Could you check a few things on this model? Use its own coordinates, in mm. A direction names the side the tool comes from. Coordinates: 2 decimals unless noted, no trailing zeros. Loops run counter-clockwise (first coordinate to the right, second up) from the corner with the lowest first, then second, coordinate; pieces in that order, holes last. Notation, with made-up numbers: M 87.25,57 L 102.25,57 A19 cw 102.25,65 Z; hole C 77.25,-36 d3. An arc over 180 degrees is marked long. Return JSON: item names as keys, results as strings. Group by question number.
from build123d import *

# Parameters (mm, degrees)
SKETCH_1_W           = 180
SKETCH_1_H           = 60
SKETCH_1_R           = 11
SKETCH_1_R_2         = 1.5
EXTRUDE_3_DEPTH      = 5
SKETCH_2_W           = 10
SKETCH_2_H           = 20
EXTRUDE_4_DEPTH      = 20
SKETCH_4_R           = 4
CUT_EXTRUDE_1_DEPTH  = 20
SKETCH_8_W           = 3
SKETCH_8_H           = 20
CUT_EXTRUDE_4_DEPTH  = 10
SKETCH_10_W          = 14
SKETCH_10_H          = 20
EXTRUDE_5_DEPTH      = 10
SKETCH_9_R           = 4
CUT_EXTRUDE_5_DEPTH  = 10
SKETCH_12_W          = 13.5
SKETCH_12_H          = 20
CUT_EXTRUDE_6_DEPTH  = 10
SKETCH_15_W          = 1
SKETCH_15_H          = 20
CUT_EXTRUDE_7_DEPTH  = 10
FILLET_5_R           = 5
SKETCH_21_W          = 10
SKETCH_21_H          = 18
EXTRUDE_6_DEPTH      = 20
SKETCH_25_W          = 11.311173877
SKETCH_25_H          = 1.5
CUT_EXTRUDE_10_DEPTH = 20
SKETCH_37_W          = 10
SKETCH_37_H          = 20
EXTRUDE_9_DEPTH      = 6
SKETCH_38_W          = 10
SKETCH_38_H          = 20
CUT_EXTRUDE_12_DEPTH = 6
SKETCH_39_R          = 4
CUT_EXTRUDE_13_DEPTH = 144.937604561
FILLET_10_R          = 8
SKETCH_41_R          = 1.5
CUT_EXTRUDE_14_DEPTH = 10
SKETCH_42_R          = 11.5
CUT_EXTRUDE_15_DEPTH = 10
SKETCH_43_R          = 1.691985253
CUT_EXTRUDE_16_DEPTH = 10
SKETCH_44_R          = 4.5
CUT_EXTRUDE_17_DEPTH = 10
CUT_EXTRUDE_18_DEPTH = 10


with BuildPart() as part:
    # 스케치1 → 보스-돌출3 (new body)
    with BuildSketch(Plane(origin=(0, 0, 0), x_dir=(1, 0, 0), z_dir=(0, 1, 0))):
        with Locations((36.632340007, -1.742375967)):
            Rectangle(SKETCH_1_W, SKETCH_1_H)
        with Locations(Location((105.632340007, 7.257624033, 0), (0, 0, 270))):
            Circle(SKETCH_1_R, mode=Mode.SUBTRACT)
        with Locations(Location((90.132340007, 22.757624033, 0), (0, 0, 270))):
            Circle(SKETCH_1_R_2, mode=Mode.SUBTRACT)
        with Locations(Location((121.132340007, 22.757624033, 0), (0, 0, 270))):
            Circle(SKETCH_1_R_2, mode=Mode.SUBTRACT)
        with Locations(Location((90.132340007, -8.242375967, 0), (0, 0, 270))):
            Circle(SKETCH_1_R_2, mode=Mode.SUBTRACT)
        with Locations(Location((121.132340007, -8.242375967, 0), (0, 0, 270))):
            Circle(SKETCH_1_R_2, mode=Mode.SUBTRACT)
        with Locations(Location((-32.617755763, 4.712595626, 0), (0, 0, 270))):
            Circle(SKETCH_1_R_2, mode=Mode.SUBTRACT)
        with Locations(Location((-45.654401225, 19.548720133, 0), (0, 0, 270))):
            Circle(SKETCH_1_R_2, mode=Mode.SUBTRACT)
        with Locations(Location((-45.654401225, -10.123528882, 0), (0, 0, 270))):
            Circle(SKETCH_1_R_2, mode=Mode.SUBTRACT)
    extrude(amount=EXTRUDE_3_DEPTH)

    # 스케치2 → 보스-돌출4 (add)
    with BuildSketch(Plane(origin=(0, 5, 0), x_dir=(1, 0, 0), z_dir=(0, 1, 0))):
        with Locations((79.782459712, 8.257624033)):
            Rectangle(SKETCH_2_W, SKETCH_2_H)
    extrude(amount=EXTRUDE_4_DEPTH)

    # 스케치4 → 컷-돌출1 (cut)
    with BuildSketch(Plane.ZY.offset(-74.782459712)):
        with Locations((-8.257624033, 15)):
            Circle(SKETCH_4_R)
    extrude(amount=-CUT_EXTRUDE_1_DEPTH, mode=Mode.SUBTRACT)

    # 스케치8 → 컷-돌출4 (cut)
    with BuildSketch(Plane(origin=(84.782459712, 0, 0), x_dir=(0, 0, -1), z_dir=(1, 0, 0))):
        with Locations((16.757624033, 15)):
            Rectangle(SKETCH_8_W, SKETCH_8_H)
        with Locations((-0.242375967, 15)):
            Rectangle(SKETCH_8_W, SKETCH_8_H)
    extrude(amount=-CUT_EXTRUDE_4_DEPTH, mode=Mode.SUBTRACT)

    # 스케치10 → 보스-돌출5 (add)
    with BuildSketch(Plane(origin=(84.782459712, 0, 0), x_dir=(0, 0, -1), z_dir=(1, 0, 0))):
        with Locations((-5.242375967, 15)):
            Rectangle(SKETCH_10_W, SKETCH_10_H)
    extrude(amount=-EXTRUDE_5_DEPTH)

    # 스케치9 → 컷-돌출5 (cut)
    with BuildSketch(Plane(origin=(84.782459712, 0, 0), x_dir=(0, 0, -1), z_dir=(1, 0, 0))):
        with Locations((-5.242375967, 15)):
            Circle(SKETCH_9_R)
    extrude(amount=-CUT_EXTRUDE_5_DEPTH, mode=Mode.SUBTRACT)

    # 스케치12 → 컷-돌출6 (cut)
    with BuildSketch(Plane(origin=(84.782459712, 0, 0), x_dir=(0, 0, -1), z_dir=(1, 0, 0))):
        with Locations((8.507624033, 15)):
            Rectangle(SKETCH_12_W, SKETCH_12_H)
    extrude(amount=-CUT_EXTRUDE_6_DEPTH, mode=Mode.SUBTRACT)

    # 스케치15 → 컷-돌출7 (cut)
    with BuildSketch(Plane(origin=(84.782459712, 0, 0), x_dir=(0, 0, -1), z_dir=(1, 0, 0))):
        with Locations((1.257624033, 15)):
            Rectangle(SKETCH_15_W, SKETCH_15_H)
    extrude(amount=-CUT_EXTRUDE_7_DEPTH, mode=Mode.SUBTRACT)

    # 필렛5
    fillet_5_edges = [part.edges().sort_by_distance(p)[0] for p in [
        (79.782459712, 25, -0.757624033),
        (79.782459712, 25, 12.242375967),
    ]]
    fillet(fillet_5_edges, radius=FILLET_5_R)

    # 스케치21 → 보스-돌출6 (add)
    with BuildSketch(Plane(origin=(0, 5, 0), x_dir=(1, 0, 0), z_dir=(0, 1, 0))):
        with Locations((79.782459712, -5.742375967)):
            Rectangle(SKETCH_21_W, SKETCH_21_H)
    extrude(amount=EXTRUDE_6_DEPTH)

    # 스케치25 → 컷-돌출10 (cut)
    with BuildSketch(Plane(origin=(0, 5, 0), x_dir=(1, 0, 0), z_dir=(0, 1, 0))):
        with Locations((79.126872773, 2.507624033)):
            Rectangle(SKETCH_25_W, SKETCH_25_H)
    extrude(amount=CUT_EXTRUDE_10_DEPTH, mode=Mode.SUBTRACT)

    # 스케치37 → 보스-돌출9 (add)
    with BuildSketch(Plane.XY.offset(14.742375967)):
        with Locations((79.782459712, 15)):
            Rectangle(SKETCH_37_W, SKETCH_37_H)
    extrude(amount=EXTRUDE_9_DEPTH)

    # 스케치38 → 컷-돌출12 (cut)
    with BuildSketch(Plane(origin=(0, 0, -1.757624033), x_dir=(-1, 0, 0), z_dir=(0, 0, -1))):
        with Locations((-79.782459712, 15)):
            Rectangle(SKETCH_38_W, SKETCH_38_H)
    extrude(amount=-CUT_EXTRUDE_12_DEPTH, mode=Mode.SUBTRACT)

    # 스케치39 → 컷-돌출13 (cut, through all)
    with BuildSketch(Plane(origin=(84.782459712, 0, 0), x_dir=(0, 0, -1), z_dir=(1, 0, 0))):
        with Locations((-11.742375967, 15)):
            Circle(SKETCH_39_R)
    extrude(amount=-CUT_EXTRUDE_13_DEPTH, mode=Mode.SUBTRACT)

    # 필렛10
    fillet_10_edges = [part.edges().sort_by_distance(p)[0] for p in [
        (79.782459712, 25, 20.742375967),
        (79.782459712, 5, 20.742375967),
        (79.782459712, 25, 4.242375967),
    ]]
    fillet(fillet_10_edges, radius=FILLET_10_R)

    # 스케치41 → 컷-돌출14 (cut)
    with BuildSketch(Plane(origin=(0, 5, 0), x_dir=(1, 0, 0), z_dir=(0, 1, 0))):
        with Locations(Location((-16.145477704, -6.751246634, 0), (0, 0, 270))):
            Circle(SKETCH_41_R)
        with Locations(Location((-16.145477704, 11.864366715, 0), (0, 0, 270))):
            Circle(SKETCH_41_R)
        with Locations(Location((0.854522296, 11.864366715, 0), (0, 0, 270))):
            Circle(SKETCH_41_R)
        with Locations(Location((0.854522296, -6.751246634, 0), (0, 0, 270))):
            Circle(SKETCH_41_R)
        with Locations(Location((17.854522296, 11.864366715, 0), (0, 0, 270))):
            Circle(SKETCH_41_R)
        with Locations(Location((17.854522296, -6.751246634, 0), (0, 0, 270))):
            Circle(SKETCH_41_R)
        with Locations(Location((34.854522296, 11.864366715, 0), (0, 0, 270))):
            Circle(SKETCH_41_R)
        with Locations(Location((34.854522296, -6.751246634, 0), (0, 0, 270))):
            Circle(SKETCH_41_R)
        with Locations(Location((51.854522296, 11.864366715, 0), (0, 0, 270))):
            Circle(SKETCH_41_R)
        with Locations(Location((51.854522296, -6.751246634, 0), (0, 0, 270))):
            Circle(SKETCH_41_R)
        with Locations(Location((68.854522296, 11.864366715, 0), (0, 0, 270))):
            Circle(SKETCH_41_R)
        with Locations(Location((68.854522296, -6.751246634, 0), (0, 0, 270))):
            Circle(SKETCH_41_R)
    extrude(amount=-CUT_EXTRUDE_14_DEPTH, mode=Mode.SUBTRACT)

    # 스케치42 → 컷-돌출15 (cut)
    with BuildSketch(Plane(origin=(0, 5, 0), x_dir=(1, 0, 0), z_dir=(0, 1, 0))):
        with Locations(Location((105.632340007, 7.257624033, 0), (0, 0, 270))):
            Circle(SKETCH_42_R)
    extrude(amount=-CUT_EXTRUDE_15_DEPTH, mode=Mode.SUBTRACT)

    # 스케치43 → 컷-돌출16 (cut)
    with BuildSketch(Plane(origin=(0, 0, 4.242375967), x_dir=(-1, 0, 0), z_dir=(0, 0, -1))):
        with Locations((-79.782459712, 14.121740896)):
            Circle(SKETCH_43_R)
    extrude(amount=-CUT_EXTRUDE_16_DEPTH, mode=Mode.SUBTRACT)

    # 스케치44 → 컷-돌출17 (cut)
    with BuildSketch(Plane.ZY.offset(-74.782459712)):
        with Locations((11.742375967, 15)):
            Circle(SKETCH_44_R)
    extrude(amount=-CUT_EXTRUDE_17_DEPTH, mode=Mode.SUBTRACT)

    # 스케치46 → 컷-돌출18 (cut)
    with BuildSketch(Plane(origin=(0, 5, 0), x_dir=(1, 0, 0), z_dir=(0, 1, 0))):
        Polygon((126.632340007, 28.257624033), (121.632340007, 28.257624033), (126.632340007, 23.257624033), align=None)
        Polygon((126.632340007, -31.742375967), (121.632340007, -31.742375967), (126.632340007, -26.742375967), align=None)
    extrude(amount=-CUT_EXTRUDE_18_DEPTH, mode=Mode.SUBTRACT)


solid = part.part
(1) If I drill on L1, parallel to X at y = 4.5, z = -8; L2, parallel to X at y = 20.5, z = 8; L3, parallel to Y at x = -38.5, z = -6, over which ranges is the centre line in solid material (lowest first)? Write a range as [from, to].
(2) We'd pull the mould along Z, two halves only. Please class faces 1 (the face through (80.15, 12.47, 5.7)), 2 (the face through (88.8, 2.46, 8.93)), 3 (the face through (79.85, 7.28, 23.15)): +Z half, -Z half, draft (parallel to the pull), parting line (faces both ways), or undercut.
(3) For faces 4 (the face through (35, 0, 1)), 5 (the face through (74.782, 13, 16)), 6 (the face through (80, 11, 4.242)), which set-ups out of +Z, -Z, +X, -X, +Y, -Y let a thin tool reach every point of the face, with its end or its side?
(4) Imagine slicing it at C-C, the plane z = -8. Write out the boundary of the cut face in (x, y), then the cut area to 3 significant figures.
(5) Imagine slicing it at A-A, the plane z = -16. Write out the boundary of the cut face in (x, y).
(6) Imagine slicing it at B-B, the plane x = 45.5. Write out the boundary of the cut face in (y, z).
(7) Will these pins go through, and if not, where does the flat tip stop? P1, Ø11.5, axis at y = 15, z = 11.74, coming from the +X side; P2, Ø5, axis at y = 8, z = 12.5, coming from the -X side; P3, Ø5, axis at x = 90.13, z = -22.76, coming from the +Y side.
Checks:
{
 "1": {"L1": "[-53.37, 94.16], [117.11, 126.63]", "L2": "[74.78, 84.78]", "L3": "[0, 5]"},
 "2": {"face 1": "draft", "face 2": "undercut", "face 3": "+Z half"},
 "3": {"face 4": "+Z, -Z, +X, -X, -Y", "face 5": "+Z, -Z, -X, +Y", "face 6": "-Z, +X, -X, +Y"},
 "4": {"outline": "M -53.37,0 L 94.16,0 L 94.16,5 L -53.37,5 Z; M 117.11,0 L 126.63,0 L 126.63,5 L 117.11,5 Z", "area": "785 mm²"},
 "5": {"outline": "M -53.37,0 L 98.16,0 L 98.16,5 L -53.37,5 Z; M 113.1,0 L 126.63,0 L 126.63,5 L 113.1,5 Z"},
 "6": {"outline": "M 0,-28.26 L 5,-28.26 L 5,31.74 L 0,31.74 Z"},
 "7": {"P1": "x = 84.78", "P2": "x = 74.78", "P3": "y = 5"}
}
